Source: CAD feature listing. Evaluate the final solid. Frame: model axes, mm. A direction names the side the tool comes from. Give positions to 0.01 mm unless a question says otherwise; leave off trailing zeros. Order: outer loops, then holes, each group sorted by start corner. A loop starts at its lowest first (then second) coordinate and runs counter-clockwise, first axis right, second up. Notation, with made-up numbers: M 28,-8 L 34,-8 A23 ccw 34,17 Z; hole C -2.5,83 d5. An arc over 180 degrees is marked long. Return JSON: item names as keys, results as strings.
from build123d import *

# Parameters (mm, degrees)
F0_R     = 2.5
F0_R_2   = 3.5
F0_R_3   = 2
F1_DEPTH = 5


with BuildPart() as f1:
    # F0 (on Front) → F1 (new body)
    with BuildSketch(Plane.XZ):
        with BuildLine():
            Line((-100, -90), (30, -90))
            Line((30, -90), (30, 10))
            ThreePointArc((30, 10), (0, 40), (-30, 10))
            Line((-30, 10), (-30, -10))
            Line((-30, -10), (-90, -10))
            ThreePointArc((-90, -10), (-97.071068, -12.928932), (-100, -20))
            Line((-100, -20), (-100, -90))
        make_face()
        with Locations((-93, -83)):
            Circle(F0_R, mode=Mode.SUBTRACT)
        with Locations((-83.2, -78.2)):
            Circle(F0_R, mode=Mode.SUBTRACT)
        with Locations((-55, -50)):
            Circle(F0_R_2, mode=Mode.SUBTRACT)
        with Locations((-26.8, -78.2)):
            Circle(F0_R, mode=Mode.SUBTRACT)
        with Locations((23, -83)):
            Circle(F0_R, mode=Mode.SUBTRACT)
        with BuildLine():
            ThreePointArc((2, -68.5), (-1.414214, -69.914214), (0, -66.5))
            ThreePointArc((0, -66.5), (1.414214, -67.085786), (2, -68.5))
        make_face(mode=Mode.SUBTRACT)
        with BuildLine():
            ThreePointArc((0, -54.25), (-4.25, -50), (0, -45.75))
            ThreePointArc((0, -45.75), (3.005204, -46.994796), (4.25, -50))
            ThreePointArc((4.25, -50), (3.005204, -53.005204), (0, -54.25))
        make_face(mode=Mode.SUBTRACT)
        with BuildLine():
            ThreePointArc((0, -33.5), (-1.414214, -30.085786), (2, -31.5))
            ThreePointArc((2, -31.5), (1.414214, -32.914214), (0, -33.5))
        make_face(mode=Mode.SUBTRACT)
        with Locations((-93, -17)):
            Circle(F0_R, mode=Mode.SUBTRACT)
        with Locations((-83.2, -21.8)):
            Circle(F0_R, mode=Mode.SUBTRACT)
        with Locations((-26.8, -21.8)):
            Circle(F0_R, mode=Mode.SUBTRACT)
        with Locations((23, -23)):
            Circle(F0_R, mode=Mode.SUBTRACT)
        with Locations((-18.5, 10)):
            Circle(F0_R_3, mode=Mode.SUBTRACT)
        with Locations((18.5, 10)):
            Circle(F0_R_3, mode=Mode.SUBTRACT)
    extrude(amount=F1_DEPTH)


solid = f1.part
1. Draft query along Z for faces 1 (the face through (-95, -2.5, -18.5)), 2 (the face through (-36, -2, -90)), 3 (the face through (-21, -5, -39)). Return one class per face: pulls with the +Z half, pulls with the -Z half, needs draft (parallel to the pull), parting line crosses it, or undercut.
Evaluation:
{"face 1": "undercut", "face 2": "pulls with the -Z half", "face 3": "needs draft"}
2. First-contact query: pin 1 (1.5 mm diameter, centred on x = 13, y = -4.5, fed in from +Z) (3 decimals); pin 2 (1.5 mm diameter, centred on y = -4, z = 22, fed in from +X); pin 3 (2 mm diameter, centred on x = -21, y = -1.5, fed in from +Z). Flat tips, straight axial feed; report the tip coordinate or a pass-through.
Evaluation:
{"pin 1": "stops at z = 37.385", "pin 2": "stops at x = 27.81", "pin 3": "stops at z = 32.36"}
3. Section query C-C (x = -26.8). Return loops of the section in (y, z), then the cut area to 3 significant figures.
Evaluation:
{"outline": "M -5,-90 L 0,-90 L 0,-80.7 L -5,-80.7 Z; M -5,-75.7 L 0,-75.7 L 0,-24.3 L -5,-24.3 Z; M -5,-19.3 L 0,-19.3 L 0,23.48 L -5,23.48 Z", "area": "517 mm^2"}
4. Section query A-A (z = -78.2). Return loops of the section in (x, y), then the cut area to 3 significant figures.
Evaluation:
{"outline": "M -100,-5 L -85.7,-5 L -85.7,0 L -100,0 Z; M -80.7,-5 L -29.3,-5 L -29.3,0 L -80.7,0 Z; M -24.3,-5 L 30,-5 L 30,0 L -24.3,0 Z", "area": "600 mm^2"}
5. Section query D-D (z = 6.5). Return loops of the section in (x, y), then the cut area to 3 significant figures.
Evaluation:
{"outline": "M -30,-5 L 30,-5 L 30,0 L -30,0 Z", "area": "300 mm^2"}
6. Set-up query: faces 4 (the face through (30, -2, -41)), 5 (the face through (-30, -2, 0)). Return all of +Z, -Z, +X, -X, +Y, -Y with unobstructed straight access to the full face (end or side cutting, diameter ignored); none if empty.
Evaluation:
{"face 4": "+Z, -Z, +X, +Y, -Y", "face 5": "+Z, -X, +Y, -Y"}
7. Ray query, probe 1 along Z at (x, y) = (-26.8, -1.85); probe 2 along Z at (x, y) = (-18.5, -3.7); probe 3 along Z at (x, y) = (-70.5, -1.45). Return the intervals inside material, ascending.
Evaluation:
{"probe 1": "z = -90 to -80.7, -75.7 to -24.3, -19.3 to 23.48", "probe 2": "z = -90 to 8, 12 to 33.62", "probe 3": "z = -90 to -10"}
8. Section query B-B (y = -2.4). State how many separate pieces and enclosed holes the cut face has, then the cut area to 3 significant figures.
Evaluation:
{"separate pieces": "1", "enclosed holes": "14", "area": "12,700 mm^2"}
